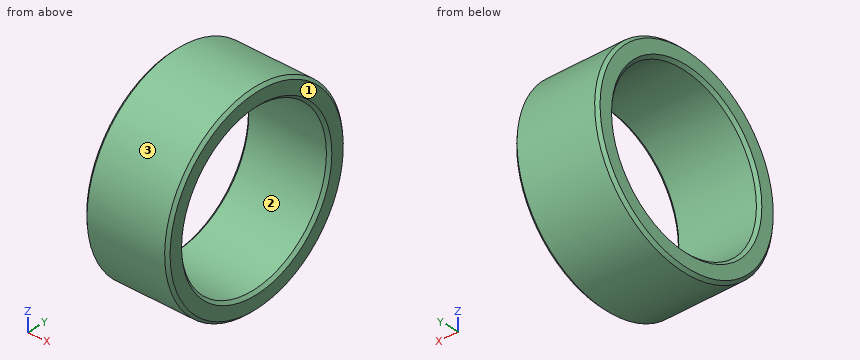
```python
from build123d import *


with BuildPart() as part:
    # Skizze1 → Rotation1 (revolve)
    with BuildSketch(Plane.XY, mode=Mode.PRIVATE) as rotation1_sk:
        Polygon((8.4, 10.5), (8.7, 10.2), (8.7, 8.85), (8.4, 8.55), (0.3, 8.55), (0, 8.85), (0, 10.2), (0.3, 10.5), align=None)
    revolve(rotation1_sk.sketch.rotate(Axis((0, 0, 0), (1, 0, 0)), 90), axis=Axis((0, 0, 0), (1, 0, 0)))


solid = part.part
```
CAD build for the part. Positions are in the model's coordinates, mm. Face numbers are marked on the shaded views. Give positions to 0.01 mm unless a question says otherwise; leave off trailing zeros. Order: outer loops, then holes, each group sorted by start corner. A loop starts at its lowest first (then second) coordinate and runs counter-clockwise, first axis right, second up. Notation, with made-up numbers: M 13,63.5 L 25,63.5 A25 cw 25,76.5 Z; hole C 29.5,73 d2. An arc over 180 degrees is marked long. Put each result on its own line as item: value. Start each with the question number.
(1) Drill centre lines: line 1 along Z through (x, y) = (5, -0.25); line 2 along Y through (x, z) = (6.5, -6.75). Where is each one in solid material? Low to high.
(2) Flat gauge pins, fed straight in: pin 1 Ø12 at (y, z) = (-3, 0) entering from -X; pin 2 Ø5 at (x, z) = (7.5, 4.5) entering from -Y; pin 3 Ø1 at (x, y) = (3.5, -2.5) entering from -Z; pin 4 Ø1 at (x, z) = (6.5, -7) entering from -Y. Where does each tip first touch, or does it go through?
(3) Saw through at A-A, the plane z = 0. Write the cut outline in (x, y).
(4) Mould opens along Z. For the marked faces 1, 2 and 3 say: +Z half, -Z half, draft (parallel to the pull), parting line (faces both ways), or undercut.
(5) Saw through at C-C, the plane x = 2.25. Write the cut outline in (y, z), then the cut area to 3 significant figures.
Check result:
1. line 1: z = -10.5 to -8.55, 8.55 to 10.5
1. line 2: y = -8.04 to -5.25, 5.25 to 8.04
2. pin 1: stops at x = 0
2. pin 2: stops at y = -10.31
2. pin 3: stops at z = -10.31
2. pin 4: stops at y = -8.25
3. outline: M 0,-10.2 L 0.3,-10.5 L 8.4,-10.5 L 8.7,-10.2 L 8.7,-8.85 L 8.4,-8.55 L 0.3,-8.55 L 0,-8.85 Z; M 0,8.85 L 0.3,8.55 L 8.4,8.55 L 8.7,8.85 L 8.7,10.2 L 8.4,10.5 L 0.3,10.5 L 0,10.2 Z
4. face 1: draft
4. face 2: undercut
4. face 3: parting line
5. outline: C 0,0 d21; hole C 0,0 d17.1
5. area: 117 mm2
